Geometry check sheet. Reference: the model listing, model coordinates, mm. Coordinates: 2 decimals unless noted, no trailing zeros. Write each loop counter-clockwise with the first axis right and the second up, starting at its lowest first coordinate (ties: lowest second). Pieces come first, ordered by that corner, then holes. Notation, with made-up numbers: (80.25, 65.25) -> (87.25, 65.25) arc R11 cw to (87.25, 79.25) -> close; hole circle Ø7 at (16, 17.5). An arc over 180 degrees is marked (long way). Use a Markdown table: item, result.
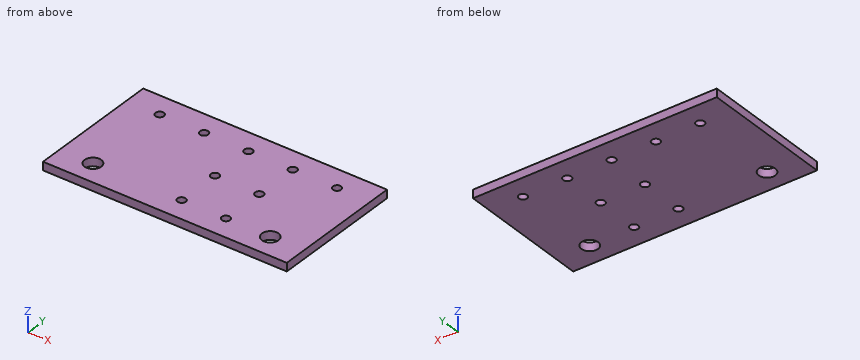
Autodesk Inventor part; units mm, degrees
ref_plane "YZ Plane" through (0, 0, 0) normal (1, 0, 0) x (0, 1, 0)
ref_plane "XZ Plane" through (0, 0, 0) normal (0, 1, 0) x (-1, 0, 0)
ref_plane "XY Plane" through (0, 0, 0) normal (0, 0, 1) x (1, 0, 0)
sketch "Sketch1" plane through (0, 0, 0) normal (0, 0, 1) x (1, 0, 0)
  line L0 (0, 0) -> (139.7, 0)
  line L1 (139.7, 0) -> (139.7, 76.2)
  line L2 (139.7, 76.2) -> (0, 76.2)
  line L3 (0, 76.2) -> (0, 0)
  dimension "d0" = 139.7
  dimension "d1" = 76.2
extrude "Extrusion1" add sketch "Sketch1" along normal blind 4.7625
sketch "Sketch2" plane through (0, 0, 4.7625) normal (0, 0, 1) x (1, 0, 0)
  line L0 (0, 0) -> (0, 76.2)
  line L1 (139.7, 0) -> (0, 0)
  circle A0 centre (19.05, 12.7) radius 4.7625
  circle A1 centre (120.65, 12.7) radius 4.7625
  line L2 (19.05, 12.7) -> (120.65, 12.7) construction
  dimension "d4" = 12.7
  dimension "d5" = 19.05
  dimension "d6" = 101.6
  dimension "d7" = 9.525
extrude "Extrusion2" cut sketch "Sketch2" against normal up to next
sketch "Sketch3" plane through (0, 0, 4.7625) normal (0, 0, 1) x (1, 0, 0)
  circle A0 centre (19.05, 12.7) radius 4.7625
  line L0 (139.7, 0) -> (0, 0)
  circle A1 centre (69.85, 12.7) radius 2.3813
  dimension "d10" = 4.7625
  dimension "d11" = 12.7
  dimension "d13" = 50.8
extrude "Extrusion3" cut sketch "Sketch3" against normal up to next contours A1
pattern_linear "Rectangular Pattern1" count 2 spacing 25.4 along (0, 1, 0) count 2 spacing 25.4 along (1, 0, 0) of "Extrusion3"
sketch "Sketch4" plane through (0, 0, 4.7625) normal (0, 0, 1) x (1, 0, 0)
  line L0 (0, 0) -> (0, 76.2)
  line L1 (0, 76.2) -> (139.7, 76.2)
  circle A0 centre (19.05, 63.5) radius 2.3813
  dimension "d22" = 4.7625
  dimension "d23" = 12.7
  dimension "d24" = 19.05
extrude "Extrusion4" cut sketch "Sketch4" against normal up to next
pattern_linear "Rectangular Pattern2" count 5 spacing 25.4 along (1, 0, 0) of "Extrusion4"
properties part number "Frame_TopFrontRollerPlate" material "Aluminum-6061"
Item 1: Depth check by flat-ended pin: P1, Ø3, axis at x = 69.85, y = 38.1, coming from the -Z side. Enter the tip coordinate at first touch or a pass-through.
Answer block:
| item | result |
|---|---|
| P1 | passes through |
Item 2: Section check B-B on x = 44.45. Record the boundary of the cut face in (y, z).
Answer block:
| item | result |
|---|---|
| outline | (0, 0) -> (61.12, 0) -> (61.12, 4.76) -> (0, 4.76) -> close; (65.88, 0) -> (76.2, 0) -> (76.2, 4.76) -> (65.88, 4.76) -> close |
Item 3: Section check D-D on y = 38.1. Record the boundary of the cut face in (x, z), then the cut area to 3 significant figures.
Answer block:
| item | result |
|---|---|
| outline | (0, 0) -> (67.47, 0) -> (67.47, 4.76) -> (0, 4.76) -> close; (72.23, 0) -> (92.87, 0) -> (92.87, 4.76) -> (72.23, 4.76) -> close; (97.63, 0) -> (139.7, 0) -> (139.7, 4.76) -> (97.63, 4.76) -> close |
| area | 620 mm^2 |
Item 4: Thickness scan on L1, parallel to Y at x = 19.05, z = 3.15; L2, parallel to Y at x = 70, z = 1.45; L3, parallel to X at y = 12.5, z = 2.5. Record the ranges inside material, lowest first. Write a range as [from, to].
Answer block:
| item | result |
|---|---|
| L1 | y = [0, 7.94], [17.46, 61.12], [65.88, 76.2] |
| L2 | y = [0, 10.32], [15.08, 35.72], [40.48, 61.12], [65.88, 76.2] |
| L3 | x = [0, 14.29], [23.81, 67.48], [72.22, 92.88], [97.62, 115.89], [125.41, 139.7] |
Item 5: Section check A-A on y = 63.5. Record the boundary of the cut face in (x, z).
Answer block:
| item | result |
|---|---|
| outline | (0, 0) -> (16.67, 0) -> (16.67, 4.76) -> (0, 4.76) -> close; (21.43, 0) -> (42.07, 0) -> (42.07, 4.76) -> (21.43, 4.76) -> close; (46.83, 0) -> (67.47, 0) -> (67.47, 4.76) -> (46.83, 4.76) -> close; (72.23, 0) -> (92.87, 0) -> (92.87, 4.76) -> (72.23, 4.76) -> close; (97.63, 0) -> (118.27, 0) -> (118.27, 4.76) -> (97.63, 4.76) -> close; (123.03, 0) -> (139.7, 0) -> (139.7, 4.76) -> (123.03, 4.76) -> close |
Item 6: Section check C-C on z = 3.6. Count the separate pieces of the cut face and the enclosed holes in it, then the cut area to 3 significant figures.
Answer block:
| item | result |
|---|---|
| separate pieces | 1 |
| enclosed holes | 11 |
| area | 10,300 mm^2 |
